from build123d import *

# Parameters (mm, degrees)
F0_W     = 38.1
F0_H     = 50.8
F1_DEPTH = 127
F2_W     = 25.4
F2_H     = 8.255
F3_DEPTH = 273.05
F5_DEPTH = 38.1
F4_R     = 12.7
F6_DEPTH = 38.1
F2_H_2   = 16.51
F7_DEPTH = 38.1


with BuildPart() as f1:
    # F0 (on Front) → F1 (new body)
    with BuildSketch(Plane.XZ):
        Polygon((0, 82.55), (0, 0), (304.8, 0), (304.8, 50.8), (266.7, 50.8), (266.7, 38.1), (31.75, 38.1), (31.75, 101.6), (19.05, 101.6), align=None)
        with Locations((285.75, 76.2)):
            Rectangle(F0_W, F0_H)
    extrude(amount=F1_DEPTH)

    # F2 (on face) → F3 (cut)
    with BuildSketch(Plane.YZ.offset(304.8)):
        with Locations((-63.5, 33.9725)):
            Rectangle(F2_W, F2_H)
        Polygon((-31.75, 29.845), (-50.8, 29.845), (-76.2, 29.845), (-95.25, 29.845), (-95.25, 16.51), (-76.2, 16.51), (-50.8, 16.51), (-31.75, 16.51), align=None)
    extrude(amount=-F3_DEPTH, mode=Mode.SUBTRACT)

    # F4 (on face) → F5 (cut, through all)
    with BuildSketch(Plane.YZ.offset(304.8)):
        with BuildLine():
            Line((0, 101.6), (-63.5, 101.6))
            ThreePointArc((-63.5, 101.6), (-51.547059, 98.611765), (-42.406574, 90.350173))
            Line((-42.406574, 90.350173), (-15.875, 50.8))
            Line((-15.875, 50.8), (0, 50.8))
            Line((0, 50.8), (0, 101.6))
        make_face()
        with BuildLine():
            Line((-127, 101.6), (-127, 50.8))
            Line((-127, 50.8), (-111.125, 50.8))
            Line((-111.125, 50.8), (-84.593426, 90.350173))
            ThreePointArc((-84.593426, 90.350173), (-75.452941, 98.611765), (-63.5, 101.6))
            Line((-63.5, 101.6), (-127, 101.6))
        make_face()
    extrude(amount=-F5_DEPTH, mode=Mode.SUBTRACT)

    # F4 (on face) → F6 (cut, through all)
    with BuildSketch(Plane.YZ.offset(304.8)):
        with Locations((-63.5, 76.2)):
            Circle(F4_R)
    extrude(amount=-F6_DEPTH, mode=Mode.SUBTRACT)

    # F2 (on face) → F7 (cut)
    with BuildSketch(Plane.YZ.offset(304.8)):
        with Locations((-63.5, 8.255)):
            Rectangle(F2_W, F2_H_2)
    extrude(amount=-F7_DEPTH, mode=Mode.SUBTRACT)


solid = f1.part
Geometry: final body of the model. Coordinates: model frame, mm. A direction names the side the tool comes from. Coordinates: 2 decimals unless noted, no trailing zeros. Order: outer loops, then holes, each group sorted by start corner. A loop starts at its lowest first (then second) coordinate and runs counter-clockwise, first axis right, second up.
1) Section A-A (x = 285). Return loops of the section in (y, z) (3 decimals), then the cut area to 3 significant figures.
Result sheet:
outline: (-127, 0) - (-76.2, 0) - (-76.2, 16.51) - (-95.25, 16.51) - (-95.25, 29.845) - (-76.2, 29.845) - (-76.2, 38.1) - (-50.8, 38.1) - (-50.8, 29.845) - (-31.75, 29.845) - (-31.75, 16.51) - (-50.8, 16.51) - (-50.8, 0) - (0, 0) - (0, 50.8) - (-15.875, 50.8) - (-42.407, 90.35) arc R25.4 ccw to (-84.593, 90.35) - (-111.125, 50.8) - (-127, 50.8) - close; hole circle Ø25.4 at (-63.5, 76.2)
area: 7,520 mm2
2) Set-up query: faces 1 (the flat face through (286, -76.2, 8)), 2 (the flat face through (170, -86, 29.845)), 3 (the flat face through (286.017, -98.045, 70.298)). Return all of +Z, -Z, +X, -X, +Y, -Y with unobstructed straight access to the full face (end or side cutting, diameter ignored); none if empty.
Result sheet:
face 1: -Z, +X
face 2: +X
face 3: +Z, +X, -Y
3) Draft query along X for faces 4 (the flat face through (9.66, -62.61, 92.21)), 5 (the flat face through (170, -76.2, 34)), 6 (the flat face through (31.75, -63, 68)). Return one class per face: released by +X, released by -X, zero draft, split by the parting line, or undercut.
Result sheet:
face 4: released by -X
face 5: zero draft
face 6: undercut
4) Section B-B (z = 76.2). Return loops of the section in (x, y), then the cut area to 3 significant figures.
Result sheet:
outline: (0, -127) - (31.75, -127) - (31.75, 0) - (0, 0) - close; (266.7, -94.09) - (304.8, -94.09) - (304.8, -76.2) - (266.7, -76.2) - close; (266.7, -50.8) - (304.8, -50.8) - (304.8, -32.91) - (266.7, -32.91) - close
area: 5,400 mm2
5) Ray query, probe 1 along Z at (x, y) = (37, -35.5) (3 decimals); probe 2 along X at (y, z) = (-27, 61); probe 3 along Z at (x, y) = (276, -63). Return the intervals inside material, ascending.
Result sheet:
probe 1: z = 0 to 16.51, 29.845 to 38.1
probe 2: x = 0 to 31.75, 266.7 to 304.8
probe 3: z = 38.1 to 63.51, 88.89 to 101.6
6) Section C-C (y = -68). Return loops of the section in (x, z).
Result sheet:
outline: (0, 0) - (266.7, 0) - (266.7, 16.51) - (31.75, 16.51) - (31.75, 101.6) - (19.05, 101.6) - (0, 82.55) - close; (266.7, 38.1) - (304.8, 38.1) - (304.8, 64.32) - (266.7, 64.32) - close; (266.7, 88.08) - (304.8, 88.08) - (304.8, 101.2) - (266.7, 101.2) - close
7) First-contact query: P1, Ø21, axis at x = 187, y = -90.5, coming from the -Z side; P2, Ø5, axis at x = 278, y = -9.5, coming from the +Z side; P3, Ø3, axis at x = 39.5, y = -86.5, coming from the +Z side; P4, Ø12.5, axis at x = 276.5, y = -67.5, coming from the -Z side. Flat tips, straight axial feed; report the tip coordinate or a pass-through.
Result sheet:
P1: stops at z = 0
P2: stops at z = 50.8
P3: stops at z = 38.1
P4: stops at z = 38.1
8) Section D-D (z = 33.5). Return loops of the section in (x, y).
Result sheet:
outline: (0, -127) - (304.8, -127) - (304.8, -76.2) - (31.75, -76.2) - (31.75, -50.8) - (304.8, -50.8) - (304.8, 0) - (0, 0) - close
